```python
from build123d import *

# Parameters (mm, degrees)
BASE_FLANGE1_DEPTH = 764
SKETCH6_R          = 10
CUT_EXTRUDE1_DEPTH = 10


# Sheet-metal steps are written as plain solids
with BuildPart() as part:
    # Sketch1 → Base-Flange1 (new body)
    with BuildSketch(Plane.XY):
        with BuildLine():
            Line((12, 0), (2, 0))
            ThreePointArc((2, 0), (0.585786438, 0.585786438), (0, 2))
            Line((0, 2), (0, 12))
            ThreePointArc((0, 12), (0.585786438, 13.414213562), (2, 14))
            Line((2, 14), (158, 14))
            ThreePointArc((158, 14), (159.414213562, 13.414213562), (160, 12))
            Line((160, 12), (160, 2))
            ThreePointArc((160, 2), (159.414213562, 0.585786438), (158, 0))
            Line((158, 0), (148, 0))
            Line((148, 0), (148, 0.8))
            Line((148, 0.8), (158, 0.8))
            ThreePointArc((158, 0.8), (158.848528137, 1.151471863), (159.2, 2))
            Line((159.2, 2), (159.2, 12))
            ThreePointArc((159.2, 12), (158.848528137, 12.848528137), (158, 13.2))
            Line((158, 13.2), (2, 13.2))
            ThreePointArc((2, 13.2), (1.151471863, 12.848528137), (0.8, 12))
            Line((0.8, 12), (0.8, 2))
            ThreePointArc((0.8, 2), (1.151471863, 1.151471863), (2, 0.8))
            Line((2, 0.8), (12, 0.8))
            Line((12, 0.8), (12, 0))
        make_face()
    extrude(amount=BASE_FLANGE1_DEPTH)

    # Sketch6 → Cut-Extrude1 (cut)
    with BuildSketch(Plane(origin=(0, 14, 0), x_dir=(1, 0, 0), z_dir=(0, 1, 0))):
        with Locations(Location((105, -299.5, 0), (0, 0, 270))):
            Circle(SKETCH6_R)
        with Locations(Location((105, -134.5, 0), (0, 0, 270))):
            Circle(SKETCH6_R)
        with Locations(Location((105, -464.5, 0), (0, 0, 270))):
            Circle(SKETCH6_R)
        with Locations(Location((105, -629.5, 0), (0, 0, 270))):
            Circle(SKETCH6_R)
        with Locations(Location((55, -629.5, 0), (0, 0, 270))):
            Circle(SKETCH6_R)
        with Locations(Location((55, -464.5, 0), (0, 0, 270))):
            Circle(SKETCH6_R)
        with Locations(Location((55, -299.5, 0), (0, 0, 270))):
            Circle(SKETCH6_R)
        with Locations(Location((55, -134.5, 0), (0, 0, 270))):
            Circle(SKETCH6_R)
    extrude(amount=-CUT_EXTRUDE1_DEPTH, mode=Mode.SUBTRACT)


solid = part.part
```
Here's how the part is built. I have some questions about the finished solid (model axes, mm). A direction names the side the tool comes from. Coordinates: 2 decimals unless noted, no trailing zeros. Order: outer loops, then holes, each group sorted by start corner. A loop starts at its lowest first (then second) coordinate and runs counter-clockwise, first axis right, second up.
1) Imagine slicing it at D-D on z = 375. List the corners of the cut face in (x, y) for me.
2) I need wall thicknesses on line 1 (X direction, y = 13.7, z = 629.5); line 2 (X direction, y = 8.5, z = 509); line 3 (Y direction, x = 10.5, z = 328). Which ranges of each line are inside material? Lowest first, please.
3) Will these pins go through, and if not, where does the flat tip stop? pin 1 (0.6 mm diameter, centred on y = 0.5, z = 319.5, fed in from -X); pin 2 (1 mm diameter, centred on x = 83, z = 506.5, fed in from -Y); pin 3 (12 mm diameter, centred on x = 55, z = 299.5, fed in from +Y).
4) Imagine slicing it at A-A on y = 4.5. List the corners of the cut face in (x, z) for me, and give its area (3 significant figures).
5) Imagine slicing it at C-C on x = 105. List the corners of the cut face in (y, z) for me.
6) We'd pull the mould along X, two halves only. Please class faces 1 (the face through (80.4, 13.8, 764)), 2 (the face through (114.915, 13.606, 133.198)), 3 (the face through (108, 13.61, 474.04)): +X half, -X half, draft (parallel to the pull), parting line (faces both ways), or undercut.
7) Imagine slicing it at B-B on z = 464.5. List the corners of the cut face in (x, y) for me.
8) Which directions (+Z, -Z, +X, -X, +Y, -Y) give clear straight access to the entire face, cutting with the end or side of a thin tool? Please do faces 4 (the face through (81, 13.2, 377)), 5 (the face through (79, 14, 377)).
Response values:
1. outline: (0, 2) arc R2 ccw to (2, 0) - (12, 0) - (12, 0.8) - (2, 0.8) arc R1.2 cw to (0.8, 2) - (0.8, 12) arc R1.2 cw to (2, 13.2) - (158, 13.2) arc R1.2 cw to (159.2, 12) - (159.2, 2) arc R1.2 cw to (158, 0.8) - (148, 0.8) - (148, 0) - (158, 0) arc R2 ccw to (160, 2) - (160, 12) arc R2 ccw to (158, 14) - (2, 14) arc R2 ccw to (0, 12) - close
2. line 1: x = 0.95 to 45, 65 to 95, 115 to 159.05
2. line 2: x = 0 to 0.8, 159.2 to 160
2. line 3: y = 0 to 0.8, 13.2 to 14
3. pin 1: stops at x = 0.4
3. pin 2: stops at y = 13.2
3. pin 3: passes through
4. outline: (0, 0) - (0.8, 0) - (0.8, 764) - (0, 764) - close; (159.2, 0) - (160, 0) - (160, 764) - (159.2, 764) - close
4. area: 1,220 mm2
5. outline: (13.2, 0) - (14, 0) - (14, 124.5) - (13.2, 124.5) - close; (13.2, 144.5) - (14, 144.5) - (14, 289.5) - (13.2, 289.5) - close; (13.2, 309.5) - (14, 309.5) - (14, 454.5) - (13.2, 454.5) - close; (13.2, 474.5) - (14, 474.5) - (14, 619.5) - (13.2, 619.5) - close; (13.2, 639.5) - (14, 639.5) - (14, 764) - (13.2, 764) - close
6. face 1: draft
6. face 2: undercut
6. face 3: undercut
7. outline: (0, 2) arc R2 ccw to (2, 0) - (12, 0) - (12, 0.8) - (2, 0.8) arc R1.2 cw to (0.8, 2) - (0.8, 12) arc R1.2 cw to (2, 13.2) - (45, 13.2) - (45, 14) - (2, 14) arc R2 ccw to (0, 12) - close; (65, 13.2) - (95, 13.2) - (95, 14) - (65, 14) - close; (115, 13.2) - (158, 13.2) arc R1.2 cw to (159.2, 12) - (159.2, 2) arc R1.2 cw to (158, 0.8) - (148, 0.8) - (148, 0) - (158, 0) arc R2 ccw to (160, 2) - (160, 12) arc R2 ccw to (158, 14) - (115, 14) - close
8. face 4: +Z, -Z
8. face 5: +Z, -Z, +X, -X, +Y
